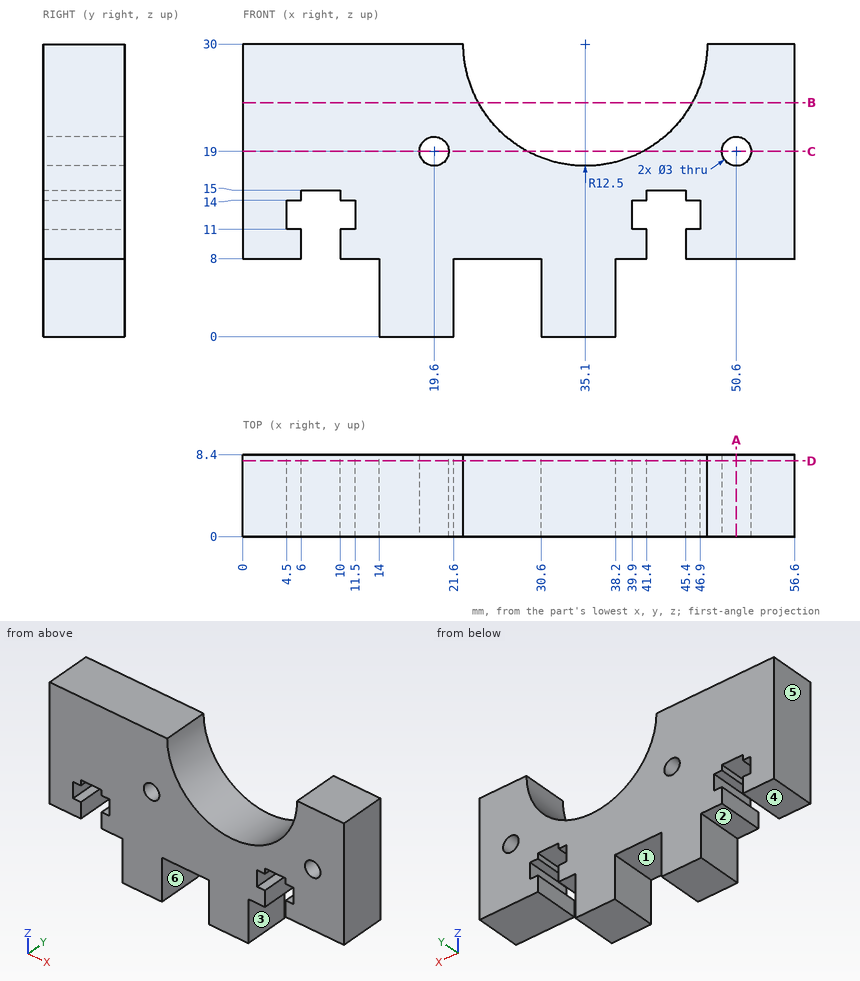
Geometry: see drawing. Coordinates: mm, zero at the bounding-box minimum. A direction names the side the tool comes from. Give positions to 0.01 mm unless a question says otherwise; leave off trailing zeros. Loops run counter-clockwise (first coordinate to the right, second up) from the corner with the lowest first, then second, coordinate; pieces in that order, holes last. Notation, with made-up numbers: (5.25, -30) - (17.25, -30) arc R13 ccw to (17.25, -20) - close; hole circle Ø7 at (75, 43). An arc over 180 degrees is marked (long way). Answer as CSV lines item,"result". Start each with the question number.
1. Section C-C, the plane z = 19. Return loops of the section in (x, y), plus the area to 3 significant figures.
2. Section D-D, the plane y = 7.75. Give the number of separate pieces and of enclosed holes in the cut face, plus the area to 3 significant figures.
3. Ray query, L1, parallel to X at y = 7.25, z = 9; L2, parallel to X at y = 8, z = 13; L3, parallel to X at y = 4.5, z = 1.5. Return the intervals inside material, ascending.
4. Pin query (flat end, axial travel): P1, Ø2.5, axis at y = 3, z = 3.5, coming from the +X side; P2, Ø4, axis at y = 5.5, z = 5, coming from the -X side; P3, Ø4, axis at x = 49, y = 6, coming from the -Z side. Return the tip coordinate at first contact, or that it passes through.
5. Reachability of the marked faces 1, 2 and 3 from +Z, -Z, +X, -X, +Y, -Y: full face, straight path, thin tool, end or side. Return the list, or none.
6. Draft query along X for the marked faces 4, 5 and 6. Return one class per face: released by +X, released by -X, zero draft, split by the parting line, or undercut.
7. Section B-B, the plane z = 24. Return loops of the section in (x, y), plus the area to 3 significant figures.
8. Section A-A, the plane x = 50.6. Return loops of the section in (y, z).
Answers:
1,outline,"(0, 0) - (18.1, 0) - (18.1, 8.4) - (0, 8.4) - close; (21.1, 0) - (29.16, 0) - (29.16, 8.4) - (21.1, 8.4) - close; (41.04, 0) - (49.1, 0) - (49.1, 8.4) - (41.04, 8.4) - close; (52.1, 0) - (56.6, 0) - (56.6, 8.4) - (52.1, 8.4) - close"
1,area,"325 mm2"
2,separate pieces,"1"
2,enclosed holes,"2"
2,area,"1,030 mm2"
3,L1,"x = 0 to 6, 10 to 41.4, 45.4 to 56.6"
3,L2,"x = 0 to 4.5, 11.5 to 39.9, 46.9 to 56.6"
3,L3,"x = 14 to 21.6, 30.6 to 38.2"
4,P1,"stops at x = 38.2"
4,P2,"stops at x = 14"
4,P3,"stops at z = 8"
5,face 1,"-Z, +Y, -Y"
5,face 2,"-Z, -X, +Y, -Y"
5,face 3,"-Z, +X, +Y, -Y"
6,face 4,"zero draft"
6,face 5,"released by -X"
6,face 6,"undercut"
7,outline,"(0, 0) - (24.13, 0) - (24.13, 8.4) - (0, 8.4) - close; (46.07, 0) - (56.6, 0) - (56.6, 8.4) - (46.07, 8.4) - close"
7,area,"291 mm2"
8,outline,"(0, 8) - (8.4, 8) - (8.4, 17.5) - (0, 17.5) - close; (0, 20.5) - (8.4, 20.5) - (8.4, 30) - (0, 30) - close"
